from build123d import *

# Parameters (mm, degrees)
SKETCH_1_R            = 2.5
SKETCH_1_W            = 7
SKETCH_1_H            = 4
EXTRUDE_1_DEPTH       = 50
HOLE_WIZARD_6_0_6_1_D = 6


with BuildPart() as part:
    # Эскиз1 → Бобышка-Вытянуть1 (new body)
    with BuildSketch(Plane(origin=(0, 0, 0), x_dir=(0, 0, -1), z_dir=(1, 0, 0))):
        with BuildLine():
            Line((-5.5, 15.8), (-5.5, 10))
            ThreePointArc((-5.5, 10), (-5.353553391, 9.646446609), (-5, 9.5))
            Line((-5, 9.5), (-0.4, 9.5))
            Line((-0.4, 9.5), (0, 9.1))
            Line((0, 9.1), (0.4, 9.5))
            Line((0.4, 9.5), (5, 9.5))
            ThreePointArc((5, 9.5), (5.353553391, 9.646446609), (5.5, 10))
            Line((5.5, 10), (5.5, 15.8))
            ThreePointArc((5.5, 15.8), (5.558578644, 15.941421356), (5.7, 16))
            Line((5.7, 16), (20.4, 16))
            ThreePointArc((20.4, 16), (20.753553391, 15.853553391), (20.9, 15.5))
            Line((20.9, 15.5), (20.9, 12.3))
            ThreePointArc((20.9, 12.3), (20.753553391, 11.946446609), (20.4, 11.8))
            Line((20.4, 11.8), (18.4, 11.8))
            ThreePointArc((18.4, 11.8), (18.258578644, 11.741421356), (18.2, 11.6))
            Line((18.2, 11.6), (18.2, 5.5))
            ThreePointArc((18.2, 5.5), (18.258578644, 5.358578644), (18.4, 5.3))
            Line((18.4, 5.3), (20.7, 5.3))
            ThreePointArc((20.7, 5.3), (20.841421356, 5.241421356), (20.9, 5.1))
            Line((20.9, 5.1), (20.9, 4.5))
            ThreePointArc((20.9, 4.5), (20.958578644, 4.358578644), (21.1, 4.3))
            Line((21.1, 4.3), (28.9, 4.3))
            ThreePointArc((28.9, 4.3), (29.041421356, 4.358578644), (29.1, 4.5))
            Line((29.1, 4.5), (29.1, 5.1))
            ThreePointArc((29.1, 5.1), (29.158578644, 5.241421356), (29.3, 5.3))
            Line((29.3, 5.3), (31.6, 5.3))
            ThreePointArc((31.6, 5.3), (31.741421356, 5.358578644), (31.8, 5.5))
            Line((31.8, 5.5), (31.8, 11.6))
            ThreePointArc((31.8, 11.6), (31.741421356, 11.741421356), (31.6, 11.8))
            Line((31.6, 11.8), (29.6, 11.8))
            ThreePointArc((29.6, 11.8), (29.246446609, 11.946446609), (29.1, 12.3))
            Line((29.1, 12.3), (29.1, 15.5))
            ThreePointArc((29.1, 15.5), (29.246446609, 15.853553391), (29.6, 16))
            Line((29.6, 16), (49.8, 16))
            ThreePointArc((49.8, 16), (49.941421356, 15.941421356), (50, 15.8))
            Line((50, 15.8), (50, 13.378675135))
            ThreePointArc((50, 13.378675135), (49.933012702, 13.128675135), (49.75, 12.945662433))
            Line((49.75, 12.945662433), (47.95, 11.906431948))
            ThreePointArc((47.95, 11.906431948), (47.766987298, 11.723419246), (47.7, 11.473419246))
            Line((47.7, 11.473419246), (47.7, 4.566580754))
            ThreePointArc((47.7, 4.566580754), (47.766987298, 4.316580754), (47.95, 4.133568052))
            Line((47.95, 4.133568052), (49.75, 3.094337567))
            ThreePointArc((49.75, 3.094337567), (49.933012702, 2.911324865), (50, 2.661324865))
            Line((50, 2.661324865), (50, 0))
            Line((50, 0), (-50, 0))
            Line((-50, 0), (-50, 2.711324865))
            ThreePointArc((-50, 2.711324865), (-50.066987298, 2.961324865), (-50.25, 3.144337567))
            Line((-50.25, 3.144337567), (-51.75, 4.010362971))
            ThreePointArc((-51.75, 4.010362971), (-51.933012702, 4.193375673), (-52, 4.443375673))
            Line((-52, 4.443375673), (-52, 11.556624327))
            ThreePointArc((-52, 11.556624327), (-51.933012702, 11.806624327), (-51.75, 11.989637029))
            Line((-51.75, 11.989637029), (-50.25, 12.855662433))
            ThreePointArc((-50.25, 12.855662433), (-50.066987298, 13.038675135), (-50, 13.288675135))
            Line((-50, 13.288675135), (-50, 15.8))
            ThreePointArc((-50, 15.8), (-49.941421356, 15.941421356), (-49.8, 16))
            Line((-49.8, 16), (-29.6, 16))
            ThreePointArc((-29.6, 16), (-29.246446609, 15.853553391), (-29.1, 15.5))
            Line((-29.1, 15.5), (-29.1, 12.3))
            ThreePointArc((-29.1, 12.3), (-29.246446609, 11.946446609), (-29.6, 11.8))
            Line((-29.6, 11.8), (-31.6, 11.8))
            ThreePointArc((-31.6, 11.8), (-31.741421356, 11.741421356), (-31.8, 11.6))
            Line((-31.8, 11.6), (-31.8, 5.5))
            ThreePointArc((-31.8, 5.5), (-31.741421356, 5.358578644), (-31.6, 5.3))
            Line((-31.6, 5.3), (-29.3, 5.3))
            ThreePointArc((-29.3, 5.3), (-29.158578644, 5.241421356), (-29.1, 5.1))
            Line((-29.1, 5.1), (-29.1, 4.5))
            ThreePointArc((-29.1, 4.5), (-29.041421356, 4.358578644), (-28.9, 4.3))
            Line((-28.9, 4.3), (-21.1, 4.3))
            ThreePointArc((-21.1, 4.3), (-20.958578644, 4.358578644), (-20.9, 4.5))
            Line((-20.9, 4.5), (-20.9, 5.1))
            ThreePointArc((-20.9, 5.1), (-20.841421356, 5.241421356), (-20.7, 5.3))
            Line((-20.7, 5.3), (-18.4, 5.3))
            ThreePointArc((-18.4, 5.3), (-18.258578644, 5.358578644), (-18.2, 5.5))
            Line((-18.2, 5.5), (-18.2, 11.6))
            ThreePointArc((-18.2, 11.6), (-18.258578644, 11.741421356), (-18.4, 11.8))
            Line((-18.4, 11.8), (-20.4, 11.8))
            ThreePointArc((-20.4, 11.8), (-20.753553391, 11.946446609), (-20.9, 12.3))
            Line((-20.9, 12.3), (-20.9, 15.5))
            ThreePointArc((-20.9, 15.5), (-20.753553391, 15.853553391), (-20.4, 16))
            Line((-20.4, 16), (-5.7, 16))
            ThreePointArc((-5.7, 16), (-5.558578644, 15.941421356), (-5.5, 15.8))
        make_face()
        with Locations((-12, 11)):
            Circle(SKETCH_1_R, mode=Mode.SUBTRACT)
        with Locations((12, 11)):
            Circle(SKETCH_1_R, mode=Mode.SUBTRACT)
        with Locations((-40, 5)):
            Circle(SKETCH_1_R, mode=Mode.SUBTRACT)
        with Locations((40, 5)):
            Circle(SKETCH_1_R, mode=Mode.SUBTRACT)
        with Locations((-11.5, 5)):
            Rectangle(SKETCH_1_W, SKETCH_1_H, mode=Mode.SUBTRACT)
        with Locations((11.5, 5)):
            Rectangle(SKETCH_1_W, SKETCH_1_H, mode=Mode.SUBTRACT)
        with BuildLine():
            Line((-45, 13), (-35, 13))
            ThreePointArc((-35, 13), (-34.646446609, 12.853553391), (-34.5, 12.5))
            Line((-34.5, 12.5), (-34.5, 9.5))
            ThreePointArc((-34.5, 9.5), (-34.646446609, 9.146446609), (-35, 9))
            Line((-35, 9), (-45, 9))
            ThreePointArc((-45, 9), (-45.353553391, 9.146446609), (-45.5, 9.5))
            Line((-45.5, 9.5), (-45.5, 12.5))
            ThreePointArc((-45.5, 12.5), (-45.353553391, 12.853553391), (-45, 13))
        make_face(mode=Mode.SUBTRACT)
        with BuildLine():
            Line((34.5, 12.5), (34.5, 9.5))
            ThreePointArc((34.5, 9.5), (34.646446609, 9.146446609), (35, 9))
            Line((35, 9), (45, 9))
            ThreePointArc((45, 9), (45.353553391, 9.146446609), (45.5, 9.5))
            Line((45.5, 9.5), (45.5, 12.5))
            ThreePointArc((45.5, 12.5), (45.353553391, 12.853553391), (45, 13))
            Line((45, 13), (35, 13))
            ThreePointArc((35, 13), (34.646446609, 12.853553391), (34.5, 12.5))
        make_face(mode=Mode.SUBTRACT)
    extrude(amount=EXTRUDE_1_DEPTH)

    # Диаметр отверстия Ø6.0 (6)1 (through all)
    with Locations(Plane(origin=(0, 4.3, 0), x_dir=(1, 0, 0), z_dir=(0, 1, 0))):
        with Locations((10, 25), (10, -25), (40, -25), (40, 25)):
            Hole(HOLE_WIZARD_6_0_6_1_D / 2)


solid = part.part
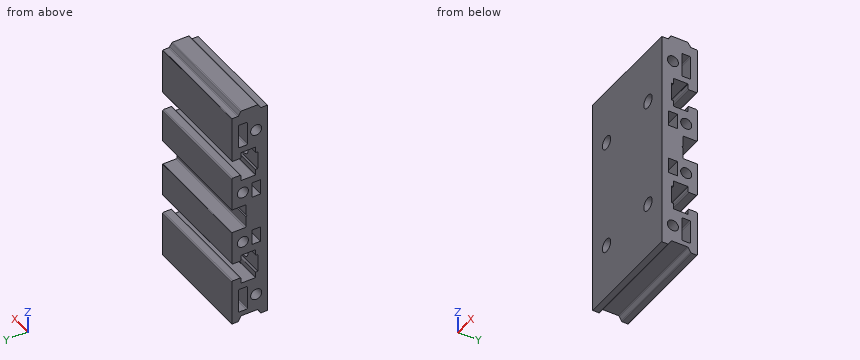
Design review of the part built by this model. Coordinates are the model's own, in mm. Coordinates: 2 decimals unless noted, no trailing zeros. Order: outer loops, then holes, each group sorted by start corner. A loop starts at its lowest first (then second) coordinate and runs counter-clockwise, first axis right, second up.
Item 1: Take a section at D-D, the plane z = 25. Write out the cut boundary in (x, y), then the cut area to 3 significant figures.
Item 2: Take a section at B-B, the plane y = 14.5. Write out the cut boundary in (x, z), then the cut area to 3 significant figures.
Item 3: For line 1 (Y direction, x = 38.5, z = 40); line 2 (Z direction, x = 16.5, y = 14.25); line 3 (X direction, y = 2.65, z = -25), list the stretches that pass through material, from the lowest coordinate up.
Item 4: Take a section at C-C, the plane x = 40. Count the separate pieces of the cut face and the enclosed holes in it, then the cut area to 3 significant figures.
Item 5: Take a section at A-A, the plane z = -40. Write out the cut boundary in (x, y).
Item 6: For pin 1 Ø3 at (x, y) = (21, 1.5) entering from +Z; pin 2 Ø3.5 at (x, y) = (18, 13.5) entering from +Z; pin 3 Ø3 at (y, z) = (11, 12) entering from -X; pin 4 Ø6.5 at (x, y) = (32.5, 9.5) entering from -Z, all flat-tipped, find the tip position at first contact; note any pin that passes through.
The answers:
1. outline: (0, 0) - (7, 0) - (7, 4.3) - (0, 4.3) - close; (13, 0) - (37, 0) - (37, 4.3) - (13, 4.3) - close; (43, 0) - (50, 0) - (50, 4.3) - (43, 4.3) - close
1. area: 163 mm2
2. outline: (0, -50) - (50, -50) - (50, -29.1) - (0, -29.1) - close; (0, -20.9) - (50, -20.9) - (50, -5.5) - (0, -5.5) - close; (0, 5.5) - (50, 5.5) - (50, 20.9) - (0, 20.9) - close; (0, 29.1) - (50, 29.1) - (50, 50) - (0, 50) - close
2. area: 3,630 mm2
3. line 1: y = 0 to 2.5, 7.5 to 9, 13 to 16
3. line 2: z = -50 to -29.1, -20.9 to -5.5, 5.5 to 20.9, 29.1 to 50
3. line 3: x = 0 to 7, 13 to 37, 43 to 50
4. separate pieces: 3
4. enclosed holes: 8
4. area: 990 mm2
5. outline: (0, 0) - (50, 0) - (50, 2.5) - (0, 2.5) - close; (0, 7.5) - (50, 7.5) - (50, 9) - (0, 9) - close; (0, 13) - (50, 13) - (50, 16) - (0, 16) - close
6. pin 1: stops at z = 50.09
6. pin 2: stops at z = 51.96
6. pin 3: passes through
6. pin 4: stops at z = -49.41
